```python
from build123d import *

# Parameters (mm, degrees)
BOSS_EXTRUDE1_DEPTH = 5.08
SKETCH2_R           = 1.5875
CUT_EXTRUDE1_DEPTH  = 50.083323044
SKETCH3_R           = 1.5875
CUT_EXTRUDE2_DEPTH  = 50.083323044
CAVITY1_START       = -1.349094449
CAVITY1_OUTLINE_R   = 1.5875
CAVITY1_DEPTH       = 5.08
CUT_EXTRUDE4_DEPTH  = 50.083323044
CAVITY3_START       = -1.147520379
CAVITY3_OUTLINE_R   = 1.5875
CAVITY3_DEPTH       = 5.08
CUT_EXTRUDE5_DEPTH  = 0.20157407


# Read off the part's stored shape, not the designer's step: Cavity1, Cavity3
with BuildPart() as part:
    # Sketch1 → Boss-Extrude1 (new body)
    with BuildSketch(Plane.XY):
        Polygon((-27.051, 40.64), (-16.891, 40.64), (-16.891, 35.56), (16.891, 35.56), (16.891, 40.64), (27.051, 40.64), (27.051, 30.48), (27.051, -40.64), (-27.051, -40.64), (-27.051, 30.48), align=None)
    extrude(amount=BOSS_EXTRUDE1_DEPTH)

    # Sketch2 → Cut-Extrude1 (cut, through all)
    with BuildSketch(Plane.XY.offset(5.08)):
        with Locations((-21.971, 38.1)):
            Circle(SKETCH2_R)
    extrude(amount=-CUT_EXTRUDE1_DEPTH, mode=Mode.SUBTRACT)

    # Sketch3 → Cut-Extrude2 (cut, through all)
    with BuildSketch(Plane(origin=(0, 0, 0), x_dir=(-1, 0, 0), z_dir=(0, 0, -1))):
        with Locations((-21.851181845, 37.741299139)):
            Circle(SKETCH3_R)
    extrude(amount=-CUT_EXTRUDE2_DEPTH, mode=Mode.SUBTRACT)

    # Cavity1 outline → Cavity1 (cut)
    with BuildSketch(Plane.YZ.offset(CAVITY1_START)):
        with BuildLine():
            Line((-14.704392822, 5.08), (-26.073978973, 5.08))
            ThreePointArc((-26.073978973, 5.08), (-25.829625006, 2.541825867), (-25.626750522, 0))
            Line((-25.626750522, 0), (-12.865436781, 0))
            ThreePointArc((-12.865436781, 0), (-13.763940636, 2.547592632), (-14.704392822, 5.08))
        make_face()
        with Locations((-18.456090827, 2.518577165)):
            Circle(CAVITY1_OUTLINE_R, mode=Mode.SUBTRACT)
    extrude(amount=CAVITY1_DEPTH, mode=Mode.SUBTRACT)

    # Sketch4 → Cut-Extrude4 (cut, through all)
    with BuildSketch(Plane.XY.offset(5.08)):
        Polygon((-3.962834865, -4.544614252), (-27.051, 25.4), (-27.051, -40.64), (27.051, -40.64), (27.051, 25.4), (6.197256749, -4.544614252), (6.197256749, -22.324614252), (3.730905551, -22.324614252), (3.730905551, -26.073978973), (-1.349094449, -26.073978973), (-1.349094449, -22.324614252), (-3.962834865, -22.324614252), align=None)
    extrude(amount=-CUT_EXTRUDE4_DEPTH, mode=Mode.SUBTRACT)


with BuildPart() as cut_extrude4_kept_piece:
    # of the separate pieces the step leaves, the one the design keeps (cut_extrude4_pieces_kept)
    add(part.part.solids().sort_by_distance((-27.051, 40.64, 0))[0])

    # Cavity3 outline → Cavity3 (cut)
    with BuildSketch(Plane.YZ.offset(CAVITY3_START)):
        with BuildLine():
            ThreePointArc((-12.347244957, 0), (-13.245748811, 2.547592632), (-14.186200998, 5.08))
            Line((-14.186200998, 5.08), (-22.324614252, 5.08))
            Line((-22.324614252, 5.08), (-22.324614252, 0))
            Line((-22.324614252, 0), (-12.347244957, 0))
        make_face()
        with Locations((-17.937899002, 2.518577165)):
            Circle(CAVITY3_OUTLINE_R, mode=Mode.SUBTRACT)
    extrude(amount=CAVITY3_DEPTH, mode=Mode.SUBTRACT)

    # Sketch7 → Cut-Extrude5 (cut)
    with BuildSketch(Plane(origin=(-1.147520379, 0, 0), x_dir=(0, 0, -1), z_dir=(1, 0, 0))):
        Polygon((-5.08, -14.186200998), (0, -12.347244957), (0, -12.865436781), (-5.08, -14.704392822), align=None)
    extrude(amount=-CUT_EXTRUDE5_DEPTH, mode=Mode.SUBTRACT)


solid = cut_extrude4_kept_piece.part
```
Here's how the part is built. I have some questions about the finished solid (model axes, mm). A direction names the side the tool comes from. Give positions to 0.01 mm unless a question says otherwise; leave off trailing zeros. Write each loop counter-clockwise with the first axis right and the second up, starting at its lowest first coordinate (ties: lowest second). Pieces come first, ordered by that corner, then holes.
(1) Thinking about a two-plate mould opening in Y: for faces 6 (the face through (5, -22.325, 3)), 7 (the face through (21.12, 36.33, 2.5)), 8 (the face through (-1.148, -19.7, 2.6)), which applies, pulls with the +Y half, pulls with the -Y half, needs draft (parallel to the pull), parting line crosses it, or undercut?
Output values:
face 6: pulls with the -Y half
face 7: undercut
face 8: needs draft
(2) Imagine slicing it at B-B, the plane x = 7.5. Write out the boundary of the cut face in (y, z), and give its area (3 significant figures).
Output values:
outline: (-2.67, 0) - (35.56, 0) - (35.56, 5.08) - (-2.67, 5.08) - close
area: 194 mm2
(3) Will these pins go through, and if not, where does the flat tip stop? pin 1 (3 mm diameter, centred on x = -1.5, z = 4, fed in from +Y); pin 2 (1 mm diameter, centred on y = 20.5, z = 2.5, fed in from -X); pin 3 (1.5 mm diameter, centred on y = -18.5, z = 2, fed in from +X); pin 4 (2.5 mm diameter, centred on x = 21.85, y = 37.74, fed in from +Z).
Output values:
pin 1: stops at y = 35.56
pin 2: stops at x = -23.66
pin 3: stops at x = 6.2
pin 4: passes through
(4) Imagine slicing it at C-C, the plane y = 14. Write out the boundary of the cut face in (x, z).
Output values:
outline: (-18.26, 0) - (19.11, 0) - (19.11, 5.08) - (-18.26, 5.08) - close
(5) On a 3-axis mill with a long thin cutter (end or side, diameter ignored), from which of +Z, -Z, +X, -X, +Y, -Y can I reach the whole of each face in a straight line? I mean faces 1 (the face through (-27.051, 33, 3)), 2 (the face through (3.731, -16.7, 2.5)), 3 (the face through (1.357, -13.233, 2.512)), 4 (the face through (-3.963, -14, 3)), 5 (the face through (-16.891, 38, 3)). Say none if no direction works.
Output values:
face 1: +Z, -Z, -X, +Y, -Y
face 2: none
face 3: -Z
face 4: +Z, -Z, -X, -Y
face 5: +Z, -Z, +Y
(6) If I drill on L1, parallel to Y at x = -21.5, z = 0.6; L2, parallel to X at y = 38, z = 4.65; L3, parallel to Y at x = 10, z = 1.75, over which ranges is the centre line in solid material (lowest first)?
Output values:
L1: y = 18.2 to 36.58, 39.62 to 40.64
L2: x = -27.05 to -23.56, -20.39 to -16.89, 16.89 to 20.28, 23.42 to 27.05
L3: y = 0.92 to 35.56
(7) Imagine slicing it at A-A, the plane x = 1.5. Write out the boundary of the cut face in (y, z) (1 decimal).
Output values:
outline: (-18.2, 1) arc R1.6 ccw to (-18.2, 4.1) arc R1.6 ccw to start; (-14.2, 5.1) arc R163.6 cw to (-12.3, 0) - (35.6, 0) - (35.6, 5.1) - close
